```python
from build123d import *

# Parameters (mm, degrees)
SKETCH1_W           = 1600
SKETCH1_H           = 650
BOSS_EXTRUDE1_DEPTH = 25
BOSS_EXTRUDE2_DEPTH = 89
SKETCH3_W           = 53
SKETCH3_H           = 50.8
BOSS_EXTRUDE3_DEPTH = 40
SKETCH4_R           = 10
CUT_EXTRUDE1_DEPTH  = 129


with BuildPart() as part:
    # Sketch1 → Boss-Extrude1 (new body)
    with BuildSketch(Plane(origin=(0, 0, 0), x_dir=(1, 0, 0), z_dir=(0, 1, 0))):
        with Locations((800, -325)):
            Rectangle(SKETCH1_W, SKETCH1_H)
    extrude(amount=BOSS_EXTRUDE1_DEPTH)

    # Sketch2 → Boss-Extrude2 (add)
    with BuildSketch(Plane.XZ):
        Polygon((38, 306), (38, 0), (0, 0), (0, 650), (38, 650), (38, 344), (1562, 344), (1562, 650), (1600, 650), (1600, 0), (1562, 0), (1562, 306), align=None)
    extrude(amount=BOSS_EXTRUDE2_DEPTH)

    # Sketch3 → Boss-Extrude3 (add)
    with BuildSketch(Plane.ZY):
        with Locations((26.5, -45.6)):
            Rectangle(SKETCH3_W, SKETCH3_H)
        with Locations((623.5, -45.6)):
            Rectangle(SKETCH3_W, SKETCH3_H)
    boss_extrude3 = extrude(amount=BOSS_EXTRUDE3_DEPTH)

    # Sketch4 → Cut-Extrude1 (cut)
    with BuildSketch(Plane.XZ.offset(71)):
        with Locations((-20, 26.5)):
            Circle(SKETCH4_R)
        with Locations((-20, 623.5)):
            Circle(SKETCH4_R)
    cut_extrude1 = extrude(amount=-CUT_EXTRUDE1_DEPTH, mode=Mode.SUBTRACT)

    # Mirror1: Boss-Extrude3, Cut-Extrude1 across plane
    add(boss_extrude3.mirror(Plane(origin=(800, 0, 0), x_dir=(0, 0, 1), z_dir=(1, 0, 0))))
    add(cut_extrude1.mirror(Plane(origin=(800, 0, 0), x_dir=(0, 0, 1), z_dir=(1, 0, 0))), mode=Mode.SUBTRACT)


solid = part.part
```
The listing builds one solid part. Answer for the finished solid, in the listing's coordinates (mm). A direction names the side the tool comes from. Round coordinates to 2 decimals unless told otherwise and drop trailing zeros. Loops run counter-clockwise (first coordinate to the right, second up) from the corner with the lowest first, then second, coordinate; pieces in that order, holes last.
Q1. Given pin 1 Ø1.5 at (x, y) = (1426.5, -28.5) entering from +Z; pin 2 Ø6 at (y, z) = (-45.5, 433.5) entering from +X; pin 3 Ø12 at (x, z) = (1345.5, 423.5) entering from -Y, each flat-ended and moving along its own axis, determine where each tip first touches the part or whether it passes through.
Q2. For a pull along X with two mould halves and no side action, classify faces 1 (the face through (-11, -71, 617)), 2 (the face through (789, 0, 495)), 3 (the face through (1640, -45, 26)) as released by +X, released by -X, zero draft, split by the parting line, or undercut.
Q3. Which of the six approach directions +Z, -Z, +X, -X, +Y, -Y give full straight-line access (tool end or side, diameter ignored) to faces 4 (the face through (789, 0, 151)), 5 (the face through (-11, -71, 20)), 6 (the face through (-11, -20.2, 20)), 7 (the face through (1611, -71, 20))?
Q4. Find the intervals of material crossed by line 1 (Z direction, x = -20, y = -56.5); line 2 (X direction, y = -59, z = 623.5); line 3 (X direction, y = -33, z = 418.5), in increasing order.
Q5. Section B-B, the plane z = 160.5 is taken. Determine the outline of the cut face in (x, y).
Q6. Section A-A, the plane y = -49 is taken. Determine the outline of the cut face in (x, z), then the cut area to 3 significant figures.
Completed:
1. pin 1: stops at z = 344
1. pin 2: stops at x = 1600
1. pin 3: stops at y = 0
2. face 1: zero draft
2. face 2: undercut
2. face 3: released by +X
3. face 4: -Z, -Y
3. face 5: +Z, -Z, -X, -Y
3. face 6: +Z, -Z, -X, +Y
3. face 7: +Z, -Z, +X, -Y
4. line 1: z = 0 to 16.5, 36.5 to 53, 597 to 613.5, 633.5 to 650
4. line 2: x = -40 to -30, -10 to 38, 1562 to 1610, 1630 to 1640
4. line 3: x = 0 to 38, 1562 to 1600
5. outline: (0, -89) - (38, -89) - (38, 0) - (1562, 0) - (1562, -89) - (1600, -89) - (1600, 25) - (0, 25) - close
6. outline: (-40, 0) - (38, 0) - (38, 306) - (1562, 306) - (1562, 0) - (1640, 0) - (1640, 53) - (1600, 53) - (1600, 597) - (1640, 597) - (1640, 650) - (1562, 650) - (1562, 344) - (38, 344) - (38, 650) - (-40, 650) - (-40, 597) - (0, 597) - (0, 53) - (-40, 53) - close; hole circle Ø20 at (-20, 26.5); hole circle Ø20 at (-20, 623.5); hole circle Ø20 at (1620, 26.5); hole circle Ø20 at (1620, 623.5)
6. area: 115,000 mm2
